Build history of the part. All positions in model axes, mm. A direction names the side the tool comes from. Round coordinates to 2 decimals unless told otherwise and drop trailing zeros. Write each loop counter-clockwise with the first axis right and the second up, starting at its lowest first coordinate (ties: lowest second). Pieces come first, ordered by that corner, then holes. Notation, with made-up numbers: (20, -36.5) -> (40, -36.5) arc R22 cw to (40, -7.5) -> close; hole circle Ø1 at (44, 48.25). An arc over 180 degrees is marked (long way). Answer in a Markdown table with one row per item.
Autodesk Inventor part; units mm, degrees
ref_plane "Work Plane1" through (8, 0, 0) normal (0, 0, -1) x (1, 0, 0)
ref_plane "YZ Plane" through (0, 0, 0) normal (1, 0, 0) x (0, 1, 0)
ref_plane "XZ Plane" through (0, 0, 0) normal (0, 1, 0) x (-1, 0, 0)
sketch "Skizze1" plane through (0, 0, 0) normal (0, 0, 1) x (1, 0, 0)
  line L0 (0, 0) -> (10, 0)
  line L1 (10, 0) -> (10, 2)
  line L2 (10, 2) -> (4, 2)
  line L3 (4, 2) -> (4, 2.75)
  line L4 (4, 2.75) -> (0, 2.75)
  line L5 (0, 2.75) -> (0, 0)
  line L6 (-2, 0) -> (12, 0)
  line L7 (0, -0.55) -> (0, 3.3)
  arc A0 (4, 2) -> (4.6, 2) centre (4.3, 2.5196) ccw
  dimension "d0" = 4
  dimension "d1" = 6
  dimension "d2" = 4
  dimension "d3" = 5.5
  dimension "d14" = 0.6
  dimension "d15" = 0.6
revolve "Körper" add sketch "Skizze1" angle 360 about axis through (0, 0, 0) along (1, 0, 0)
sketch "Skizze2" plane through (0, 0, 0) normal (-1, 0, 0) x (0, 0, 1)
  circle A0 centre (0, 0) radius 2.75
  line L0 (0, -3.85) -> (0, 3.85)
  line L1 (-3.85, 0) -> (3.85, 0)
  line L2 (-2.75, 0.3) -> (2.75, 0.3)
  line L3 (2.75, 0.3) -> (2.75, -0.3)
  line L4 (2.75, -0.3) -> (-2.75, -0.3)
  line L5 (-2.75, -0.3) -> (-2.75, 0.3)
  line L6 (-2.75, 0) -> (2.75, 0) construction
  line L7 (0, 0.3) -> (0, -0.3) construction
  dimension "d5" = 0.6
extrude "Loch" cut sketch "Skizze2" against normal blind 1.42 contours L1 L0 L2 A0 | L3 L4 A0 | A0 L4 L0 L1 | A0 L2 L3 | L1 A0 L2 L0 | L0 L4 A0 L1 | L5 L2 A0 | A0 L4 L5
chamfer "Fase1" distance 0.8 angle 45 3 edges at (0, 2.0479, -1.8354) (0, 2.0479, 1.8354) (0, -2.75, 0) measured on face at (1.8067, 0.7465, 2.6467)
thread "Gewinde"
chamfer "Fase2" distance 0.4294 distance2 0.4294 1 edges at (10, -2, 0) measured on face at (10, -0.499, -0.4421)
revolve "Nut1" cut sketch "Skizze1" angle 360 about axis through (0, 0, 0) along (1, 0, 0) contours A0 L2
ref_plane "Work Plane1" through (8, 0, 0) normal (0, 0, -1) x (1, 0, 0)
equation "\"d0\" = KOH"
equation "\"d1\" = GEL"
equation "\"d2\" = NND"
equation "\"d3\" = KOD"
equation "\"d14\" = SBR"
equation "\"d15\" = SBR"
equation "\"d5\" = SBR"
equation "\"d6\" = STI"
equation "\"d8\" = PHH"
equation "\"d19\" = PHH"
equation "\"d10\" = GEL"
equation "\"d12\" = -0.5 * GD1 + 0.5 * NND"
equation "\"d13\" = GUL"
equation "\"NND\" = 4"
equation "\"GEL\" = 6"
equation "\"KOD\" = 5.5"
equation "\"KOH\" = 4"
equation "\"SBR\" = 0.6"
equation "\"GUL\" = 0.61345 * PTC"
equation "\"PHH\" = 0.8"
equation "\"GD1\" = THREADDIA - 1.2269 * PTC"
equation "\"STI\" = 1.42"
equation "\"THREADDIA\" = 4"
equation "\"TOA\" = 30deg"
equation "\"NLG\" = GEL"
equation "\"PTC\" = 0.7"
equation "\"GAL\" = 0.61345 * PTC"
properties part number "DIN 927 - M4 x 4-14H" material "Stahl, weich"
Q1. Drop flat-ended pins along their axis: P1, Ø0.7, axis at x = 0.5, z = -0.5, coming from the -Y side; P2, Ø0.7, axis at x = 1, z = 1, coming from the +Y side; P3, Ø1.5, axis at x = 6, y = 0, coming from the -Z side. Give the stop position or say it passes through.
A:
| item | result |
|---|---|
| P1 | y = -2.73 |
| P2 | y = 2.67 |
| P3 | z = -2 |
Q2. Two-plate mould, pull along Y, no slides. Class faces 1 (the flat face through (1, 0.3, 0)), 2 (the flat face through (4, 1, -2)), 3 (the flat face through (1, -0.3, 0)), 4 (the conical face through (0.14, -2.09, 0.04)): released by +Y, released by -Y, zero draft, split by the parting line, or undercut.
A:
| item | result |
|---|---|
| face 1 | undercut |
| face 2 | zero draft |
| face 3 | undercut |
| face 4 | released by -Y |
Q3. Which spindle directions (+Z, -Z, +X, -X, +Y, -Y) get a long thin tool onto all of the face, cutting with end or side? Do faces 5 (the cylindrical face through (7, 0, 2)), 6 (the conical face through (0.14, 2.09, -0.04)). Say none if no direction does.
A:
| item | result |
|---|---|
| face 5 | +X |
| face 6 | -X, +Y |
Q4. Saw through at A-A on y = 0. Write the cut outline in (x, z), plus the area to 3 significant figures.
A:
| item | result |
|---|---|
| outline | (1.42, -2.75) -> (4, -2.75) -> (4, -2) arc R0.6 cw to (4.6, -2) -> (9.57, -2) -> (10, -1.57) -> (10, 1.57) -> (9.57, 2) -> (4.6, 2) arc R0.6 cw to (4, 2) -> (4, 2.75) -> (1.42, 2.75) -> close |
| area | 37.9 mm² |
Q5. Saw through at D-D on x = 6.75. Write the cut outline in (y, z), plus the area to 3 significant figures.
A:
| item | result |
|---|---|
| outline | circle Ø4 at (0, 0) |
| area | 12.6 mm² |
Q6. Saw through at B-B on z = 0. Write the cut outline in (x, y), plus the area to 3 significant figures.
A:
| item | result |
|---|---|
| outline | (0, -1.95) -> (0.8, -2.75) -> (4, -2.75) -> (4, -2) arc R0.6 cw to (4.6, -2) -> (9.57, -2) -> (10, -1.57) -> (10, 1.57) -> (9.57, 2) -> (4.6, 2) arc R0.6 cw to (4, 2) -> (4, 2.75) -> (0.8, 2.75) -> (0, 1.95) -> (0, 0.3) -> (1.42, 0.3) -> (1.42, -0.3) -> (0, -0.3) -> close |
| area | 44.3 mm² |
Q7. Wall check: line 1 (X direction, y = 0.15, z = 1.5); line 2 (Z direction, x = 1.75, y = -0.3); line 3 (Z direction, x = 8, y = -0.1). Give the ranges that are in metal, low to high. Write a range as [from, to].
A:
| item | result |
|---|---|
| line 1 | [1.42, 10] |
| line 2 | [-2.73, 2.73] |
| line 3 | [-2, 2] |
